from build123d import *

# Parameters (mm, degrees)
SKETCH1_R           = 17.5
SKETCH1_R_2         = 2.5
SKETCH1_R_3         = 4
BOSS_EXTRUDE1_DEPTH = 4
SKETCH3_R           = 4
BOSS_EXTRUDE2_DEPTH = 10
SKETCH4_R           = 2.45
CUT_EXTRUDE1_DEPTH  = 4


with BuildPart() as part:
    # Sketch1 → Boss-Extrude1 (new body)
    with BuildSketch(Plane.XY):
        Circle(SKETCH1_R)
        with Locations((0, 12)):
            Circle(SKETCH1_R_2, mode=Mode.SUBTRACT)
        with Locations((10.392304845, 6)):
            Circle(SKETCH1_R_2, mode=Mode.SUBTRACT)
        with Locations((10.392304845, -6)):
            Circle(SKETCH1_R_2, mode=Mode.SUBTRACT)
        with Locations((0, -12)):
            Circle(SKETCH1_R_2, mode=Mode.SUBTRACT)
        with Locations((-10.392304845, -6)):
            Circle(SKETCH1_R_2, mode=Mode.SUBTRACT)
        with Locations((-10.392304845, 6)):
            Circle(SKETCH1_R_2, mode=Mode.SUBTRACT)
        Circle(SKETCH1_R_3, mode=Mode.SUBTRACT)
    extrude(amount=BOSS_EXTRUDE1_DEPTH)

    # Sketch3 → Boss-Extrude2 (add)
    with BuildSketch(Plane.XY.offset(4)):
        with BuildLine():
            Line((2.355105774, 6.591925121), (-2.355105774, 6.591925121))
            ThreePointArc((-2.355105774, 6.591925121), (0, -7), (2.355105774, 6.591925121))
        make_face()
        Circle(SKETCH3_R, mode=Mode.SUBTRACT)
    extrude(amount=BOSS_EXTRUDE2_DEPTH)

    # Sketch4 → Cut-Extrude1 (cut)
    with BuildSketch(Plane(origin=(0, 6.591925121, 0), x_dir=(1, 0, 0), z_dir=(0, 1, 0))):
        with Locations(Location((0, -9, 0), (0, 0, 270))):
            Circle(SKETCH4_R)
    extrude(amount=-CUT_EXTRUDE1_DEPTH, mode=Mode.SUBTRACT)


solid = part.part
Read the model definition and answer for the solid it produces. Units are mm, in the model's axes. A direction names the side the tool comes from. Round coordinates to 2 decimals unless told otherwise and drop trailing zeros. Write each loop counter-clockwise with the first axis right and the second up, starting at its lowest first coordinate (ties: lowest second). Pieces come first, ordered by that corner, then holes.
1. The part is cut by section C-C, the plane z = 3.5. Determine the outline of the cut face in (x, y).
2. Determine the mould class of faces 5 (the face through (-0.54, 9.56, 1.97)), 6 (the face through (-13.887, -10.648, 1.972)), 7 (the face through (4, -4, 0)) for opening direction Y: pulls with the +Y half, pulls with the -Y half, needs draft (parallel to the pull), parting line crosses it, or undercut.
3. Straight lines are drawn through the part: L1, parallel to Z at x = -7.5, y = -9; L2, parallel to Z at x = 0, y = 5.5; L3, parallel to X at y = 5, z = 7.25. For each, find the intervals that lie inside material, in ascending order.
4. The part is cut by section B-B, the plane x = 3.5. Determine the outline of the cut face in (y, z), then the cut area to 3 significant figures.
5. The part is cut by section D-D, the plane y = 6. Determine the outline of the cut face in (x, z).
6. Given pin 1 Ø5 at (x, y) = (0, 0) entering from -Z; pin 2 Ø2 at (x, z) = (0, 12.5) entering from +Y; pin 3 Ø6 at (y, z) = (-11.5, 2) entering from -X; pin 4 Ø4 at (x, z) = (9, 5.5) entering from +Y, each flat-ended and moving along its own axis, determine where each tip first touches the part or whether it passes through.
7. The part is cut by section A-A, the plane y = 0. Determine the outline of the cut face in (x, z).
8. Which of the six approach directions +Z, -Z, +X, -X, +Y, -Y give full straight-line access (tool end or side, diameter ignored) to faces 1 (the face through (0, -8, 4)), 2 (the face through (-1.491, 4.901, 7.056)), 3 (the face through (-12.89, 6.11, 1.97)), 4 (the face through (0, 6.592, 12))?
Values:
1. outline: circle Ø35 at (0, 0); hole circle Ø5 at (-10.39, -6); hole circle Ø5 at (-10.39, 6); hole circle Ø8 at (0, 0); hole circle Ø5 at (0, -12); hole circle Ø5 at (0, 12); hole circle Ø5 at (10.39, -6); hole circle Ø5 at (10.39, 6)
2. face 5: undercut
2. face 6: parting line crosses it
2. face 7: needs draft
3. L1: z = 0 to 4
3. L2: z = 0 to 6.55, 11.45 to 14
3. L3: x = -4.9 to -1.71, 1.71 to 4.9
4. outline: (-17.15, 0) - (-1.94, 0) - (-1.94, 14) - (-6.06, 14) - (-6.06, 4) - (-17.15, 4) - close; (1.94, 0) - (17.15, 0) - (17.15, 4) - (6.06, 4) - (6.06, 14) - (1.94, 14) - close
4. area: 204 mm2
5. outline: (-16.44, 0) - (-12.89, 0) - (-12.89, 4) - (-16.44, 4) - close; (-7.89, 0) - (7.89, 0) - (7.89, 4) - (3.61, 4) - (3.61, 14) - (-3.61, 14) - (-3.61, 4) - (-7.89, 4) - close; (12.89, 0) - (16.44, 0) - (16.44, 4) - (12.89, 4) - close; hole circle Ø4.9 at (0, 9)
6. pin 1: passes through
6. pin 2: stops at y = 6.59
6. pin 3: stops at x = -15.3
6. pin 4: stops at y = 15.73
7. outline: (-17.5, 0) - (-4, 0) - (-4, 14) - (-7, 14) - (-7, 4) - (-17.5, 4) - close; (4, 0) - (17.5, 0) - (17.5, 4) - (7, 4) - (7, 14) - (4, 14) - close
8. face 1: +Z
8. face 2: +Y
8. face 3: +Z, -Z
8. face 4: +Z, +X, -X, +Y
